Work out the finished part from the listing and answer in its coordinate system (mm). Give positions to 0.01 mm unless a question says otherwise; leave off trailing zeros. Order: outer loops, then holes, each group sorted by start corner. A loop starts at its lowest first (then second) coordinate and runs counter-clockwise, first axis right, second up.
```python
from build123d import *

# Parameters (mm, degrees)
F0_R     = 4.7625
F1_DEPTH = 6.35


with BuildPart() as f1:
    # F0 (on Top) → F1 (new body)
    with BuildSketch(Plane.XY):
        with BuildLine():
            Line((-269.875, 0), (0, -269.875))
            ThreePointArc((0, -269.875), (191.033844, 191.033844), (-269.875, 0))
        make_face()
        with Locations((-124.610205, -124.610205)):
            Circle(F0_R, mode=Mode.SUBTRACT)
        with BuildLine():
            ThreePointArc((16.784284, 9.010566), (18.47489, 4.645529), (19.05, 0))
            ThreePointArc((19.05, 0), (-16.348605, -9.778835), (9.010566, 16.784284))
            ThreePointArc((9.010566, 16.784284), (15.21567, 18.745409), (19.026634, 13.470384))
            ThreePointArc((19.026634, 13.470384), (18.434494, 10.974482), (16.784284, 9.010566))
        make_face(mode=Mode.SUBTRACT)
        with Locations((41.622845, -251.873195)):
            Circle(F0_R, mode=Mode.SUBTRACT)
        with Locations((181.720938, -179.304401)):
            Circle(F0_R, mode=Mode.SUBTRACT)
        with Locations((252.40781, -38.24742)):
            Circle(F0_R, mode=Mode.SUBTRACT)
        with Locations((-252.40781, 38.24742)):
            Circle(F0_R, mode=Mode.SUBTRACT)
        with Locations((-181.720938, 179.304401)):
            Circle(F0_R, mode=Mode.SUBTRACT)
        with Locations((-41.622845, 251.873195)):
            Circle(F0_R, mode=Mode.SUBTRACT)
        with Locations((226.683477, 117.418776)):
            Circle(F0_R, mode=Mode.SUBTRACT)
    extrude(amount=-F1_DEPTH)


solid = f1.part
```
1. The part is cut by section C-C (y = 156.5). Write down the section's boundary in (x, z).
Findings below:
outline: (-219.98, -6.35) - (220.21, -6.35) - (220.21, 0) - (-219.98, 0) - close
2. The part is cut by section A-A (z = -1). State how many separate pieces and enclosed holes the cut face has, then the cut area to 3 significant figures.
Findings below:
separate pieces: 1
enclosed holes: 9
area: 206,000 mm2
3. The part is cut by section B-B (x = 208). Write down the section's boundary in (y, z), then the cut area to 3 significant figures.
Findings below:
outline: (-172.17, -6.35) - (172.4, -6.35) - (172.4, 0) - (-172.17, 0) - close
area: 2,190 mm2
4. Given P1, Ø8.5, axis at x = -252.41, y = 38.25, coming from the -Z side; P2, Ø5, axis at x = -36, y = 28, coming from the +Z side; P3, Ø1.5, axis at y = 115.5, z = -5.5, coming from the +X side, each flat-ended and moving along its own axis, determine where each tip first touches the part or whether it passes through.
Findings below:
P1: passes through
P2: stops at z = 0
P3: stops at x = 244.57
5. Straight lines are drawn through the part: probe 1 along Y at (x, z) = (45, -4.75); probe 2 along Y at (x, z) = (-179.5, -2.25) (3 decimals); probe 3 along X at (y, z) = (84, -3.5). For each, find the intervals that lie inside material, in ascending order.
Findings below:
probe 1: y = -266.12 to -255.23, -248.52 to 266.36
probe 2: y = -90.375 to 175.091, 183.517 to 201.697
probe 3: x = -256.51 to 256.75
